Check sheet for the drawn part. Datum: minimum x, y, z corner. Units: mm. Coordinates: 2 decimals unless noted, no trailing zeros. Order: outer loops, then holes, each group sorted by start corner. A loop starts at its lowest first (then second) coordinate and runs counter-clockwise, first axis right, second up. Notation, with made-up numbers: (-36.75, 49) -> (0.25, 49) arc R7 ccw to (0.25, 59) -> close; hole circle Ø6 at (-10.5, 85.5). An arc over 180 degrees is marked (long way). Answer as CSV lines item,"result".
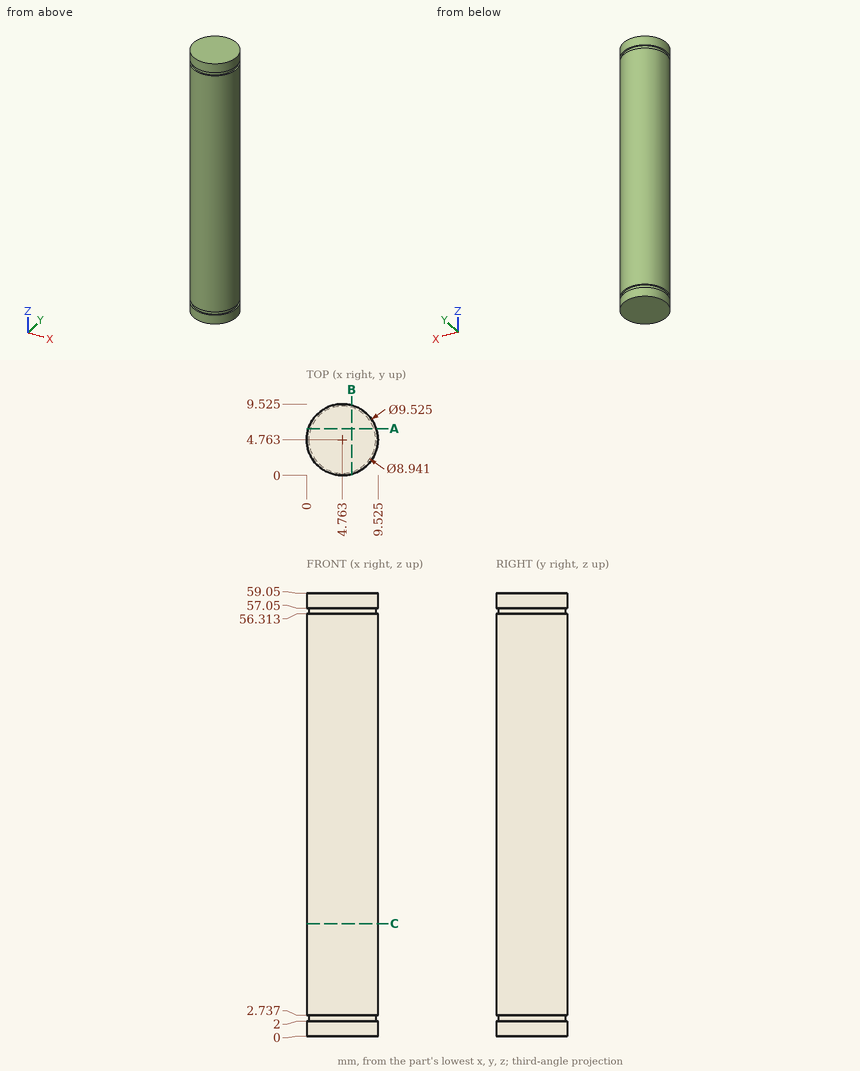
Item 1: Thickness scan on line 1 (Z direction, x = 2.75, y = 0.5); line 2 (X direction, y = 5, z = 43.5) (1 decimal); line 3 (Y direction, x = 6.5, z = 42) (1 decimal). Record the ranges inside material, lowest first.
Answer list:
line 1,"0 to 2, 2.74 to 56.31, 57.05 to 59.05"
line 2,"0 to 9.5"
line 3,"0.3 to 9.2"
Item 2: Section check A-A, the plane y = 6.25. Record the boundary of the cut face in (x, z).
Answer list:
outline,"(0.24, 0) -> (9.29, 0) -> (9.29, 2) -> (8.98, 2) -> (8.98, 2.74) -> (9.29, 2.74) -> (9.29, 56.31) -> (8.98, 56.31) -> (8.98, 57.05) -> (9.29, 57.05) -> (9.29, 59.05) -> (0.24, 59.05) -> (0.24, 57.05) -> (0.55, 57.05) -> (0.55, 56.31) -> (0.24, 56.31) -> (0.24, 2.74) -> (0.55, 2.74) -> (0.55, 2) -> (0.24, 2) -> close"
Item 3: Section check B-B, the plane x = 6. Record the boundary of the cut face in (y, z).
Answer list:
outline,"(0.16, 0) -> (9.36, 0) -> (9.36, 2) -> (9.06, 2) -> (9.06, 2.74) -> (9.36, 2.74) -> (9.36, 56.31) -> (9.06, 56.31) -> (9.06, 57.05) -> (9.36, 57.05) -> (9.36, 59.05) -> (0.16, 59.05) -> (0.16, 57.05) -> (0.47, 57.05) -> (0.47, 56.31) -> (0.16, 56.31) -> (0.16, 2.74) -> (0.47, 2.74) -> (0.47, 2) -> (0.16, 2) -> close"
Item 4: Section check C-C, the plane z = 15. Record the boundary of the cut face in (x, y) (1 decimal).
Answer list:
outline,"circle Ø9.5 at (4.8, 4.8)"
Item 5: Depth check by flat-ended pin: pin 1 Ø2 at (y, z) = (8.5, 50.5) entering from -X (1 decimal); pin 2 Ø2 at (x, z) = (1.5, 33.5) entering from +Y; pin 3 Ø2 at (x, z) = (3, 37) entering from -Y. Enter the tip coordinate at first touch or a pass-through.
Answer list:
pin 1,"x = 0.9"
pin 2,"y = 8.95"
pin 3,"y = 0.06"
